For this review, use the dimensioned drawing (mm, ordinates from the lowest corner) and the shaded views. Round coordinates to 2 decimals unless told otherwise and drop trailing zeros. Loops run counter-clockwise (first coordinate to the right, second up) from the corner with the lowest first, then second, coordinate; pieces in that order, holes last. Notation, with made-up numbers: M 23,1 L 41,1 A16 cw 41,7 Z; hole C 26.5,63 d5. An arc over 180 degrees is marked long. One line per item, written item: value. Start each with the question number.
Item 1: We need section D-D (z = 55). Write out the cut boundary in (x, y), then the cut area to 3 significant figures.
Item 2: For line 1 along X through (y, z) = (4.75, 97); line 2 along X through (y, z) = (3, 55); line 3 along X through (y, z) = (7, 96), list the stretches that pass through material, from the lowest coordinate up.
Item 3: We need section A-A (z = 97). Write out the cut boundary in (x, y).
Item 4: We need section B-B (x = 13). Write out the cut boundary in (y, z), then the cut area to 3 significant figures.
Item 5: We need section C-C (x = 55). Write out the cut boundary in (y, z).
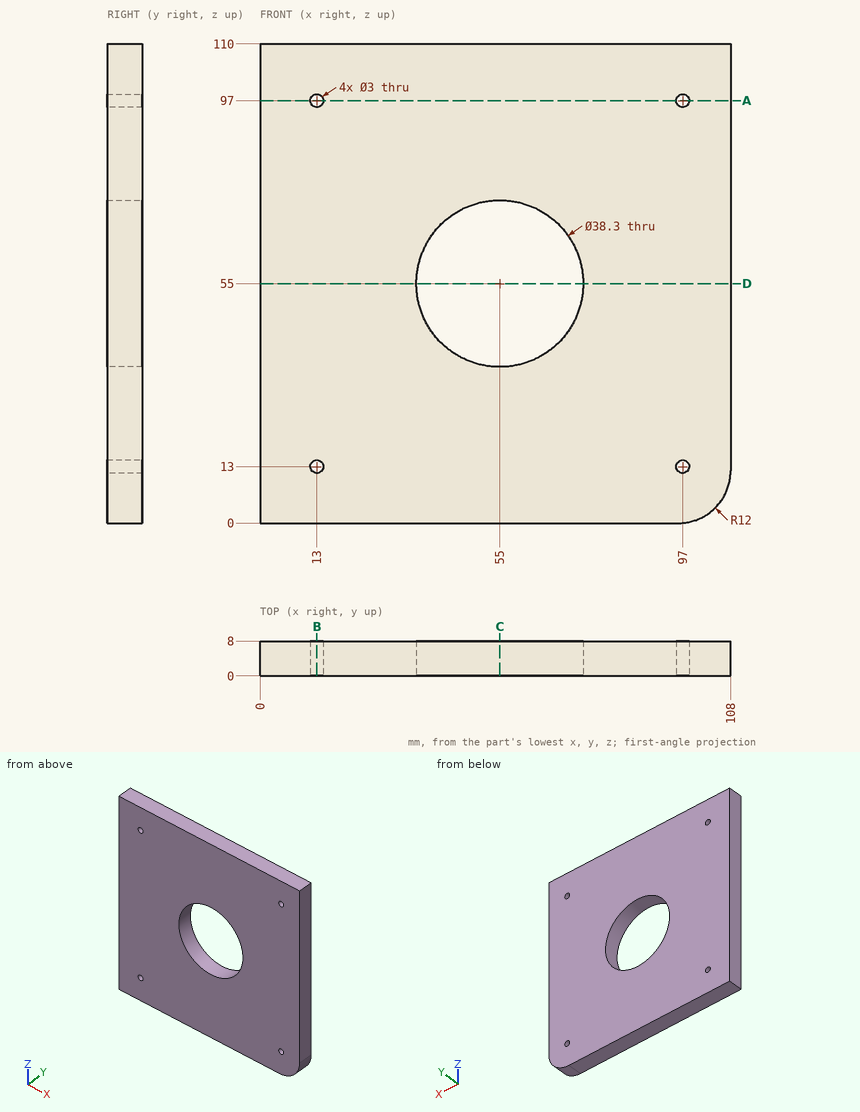
A:
1. outline: M 0,0 L 35.85,0 L 35.85,8 L 0,8 Z; M 74.15,0 L 108,0 L 108,8 L 74.15,8 Z
1. area: 558 mm2
2. line 1: 0 to 11.5, 14.5 to 95.5, 98.5 to 108
2. line 2: 0 to 35.85, 74.15 to 108
2. line 3: 0 to 11.88, 14.12 to 95.88, 98.12 to 108
3. outline: M 0,0 L 11.5,0 L 11.5,8 L 0,8 Z; M 14.5,0 L 95.5,0 L 95.5,8 L 14.5,8 Z; M 98.5,0 L 108,0 L 108,8 L 98.5,8 Z
4. outline: M 0,0 L 8,0 L 8,11.5 L 0,11.5 Z; M 0,14.5 L 8,14.5 L 8,95.5 L 0,95.5 Z; M 0,98.5 L 8,98.5 L 8,110 L 0,110 Z
4. area: 832 mm2
5. outline: M 0,0 L 8,0 L 8,35.85 L 0,35.85 Z; M 0,74.15 L 8,74.15 L 8,110 L 0,110 Z
